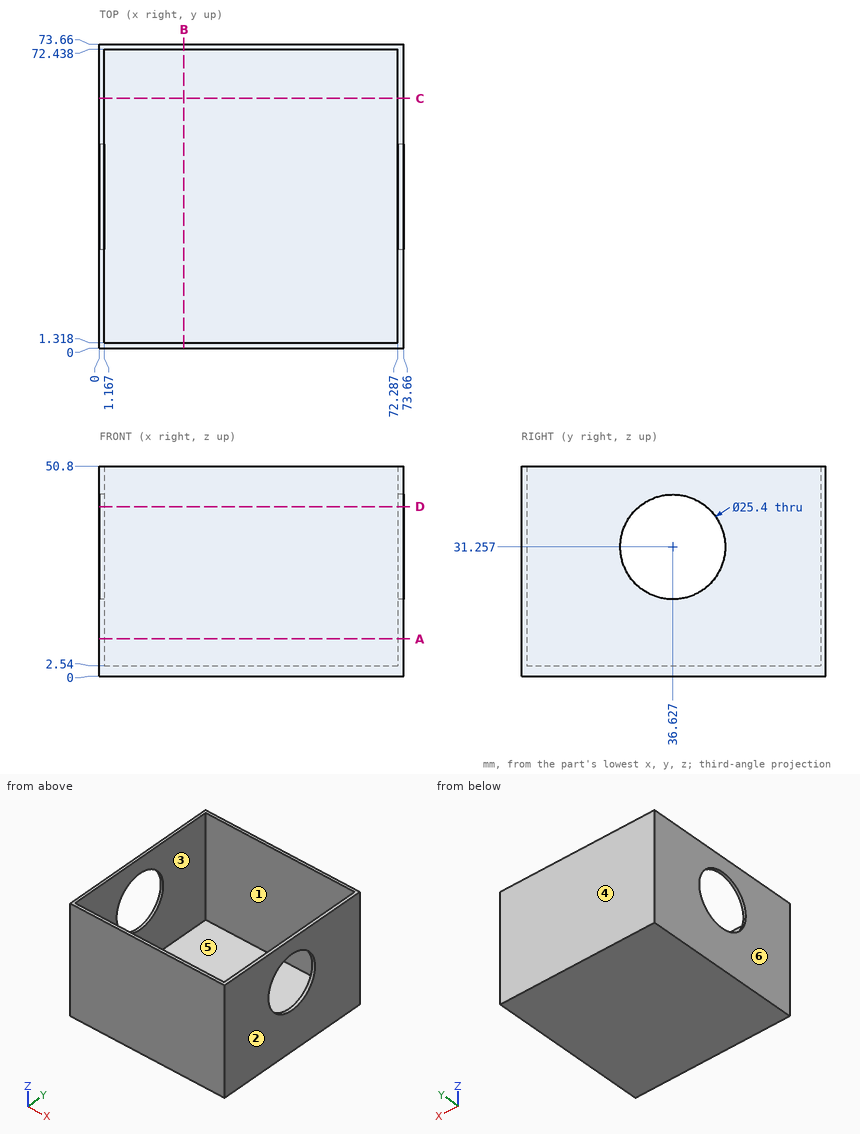
Drawing for the job (mm, zero at the part's lowest x, y, z). A direction names the side the tool comes from. Round coordinates to 2 decimals unless told otherwise and drop trailing zeros. Write each loop counter-clockwise with the first axis right and the second up, starting at its lowest first coordinate (ties: lowest second). Pieces come first, ordered by that corner, then holes. Notation, with made-up numbers: (4.5, 59.25) - (40.5, 59.25) arc R21 cw to (40.5, 79.25) - close; hole circle Ø11 at (67, 29). An arc over 180 degrees is marked (long way). Return JSON: item names as keys, results as strings. Group by question number.
Item 1: Band-saw the part on A-A on z = 9. List the corners of the cut face in (x, y).
Item 2: Flat gauge pin, fed straight in: pin 1 Ø4 at (x, y) = (31.5, 60.5) entering from +Z. Where does the tip first touch, or does it go through?
Item 3: Mould opens along Y. For the marked faces 1, 2, 3 and 4 say: +Y half, -Y half, draft (parallel to the pull), parting line (faces both ways), or undercut.
Item 4: Band-saw the part on D-D on z = 41. List the corners of the cut face in (x, y).
Item 5: Band-saw the part on B-B on x = 20.5. List the corners of the cut face in (y, z).
Item 6: 3-axis set-ups, long thin cutter, end or side, ignore diameter. For the marked faces 5 and 6: which of +Z, -Z, +X, -X, +Y, -Y reach the whole face in a straight line?
Item 7: Band-saw the part on C-C on y = 60.5. List the corners of the cut face in (x, z).
Item 8: Probe probe 1 along X at (y, z) = (44, 4); probe 2 along Y at (x, z) = (68, 37.5); probe 3 along Z at (x, y) = (69, 27). List the from-to ranges inside material, lowest first.
Resolved:
{
 "1": {"outline": "(0, 0) - (73.66, 0) - (73.66, 73.66) - (0, 73.66) - close; hole (1.17, 1.32) - (72.29, 1.32) - (72.29, 72.44) - (1.17, 72.44) - close"},
 "2": {"pin 1": "stops at z = 2.54"},
 "3": {"face 1": "undercut", "face 2": "draft", "face 3": "undercut", "face 4": "+Y half"},
 "4": {"outline": "(0, 0) - (73.66, 0) - (73.66, 28.48) - (72.29, 28.48) - (72.29, 1.32) - (1.17, 1.32) - (1.17, 28.48) - (0, 28.48) - close; (0, 44.77) - (1.17, 44.77) - (1.17, 72.44) - (72.29, 72.44) - (72.29, 44.77) - (73.66, 44.77) - (73.66, 73.66) - (0, 73.66) - close"},
 "5": {"outline": "(0, 0) - (73.66, 0) - (73.66, 50.8) - (72.44, 50.8) - (72.44, 2.54) - (1.32, 2.54) - (1.32, 50.8) - (0, 50.8) - close"},
 "6": {"face 5": "+Z", "face 6": "+Z, -Z, -X, +Y, -Y"},
 "7": {"outline": "(0, 0) - (73.66, 0) - (73.66, 50.8) - (72.29, 50.8) - (72.29, 2.54) - (1.17, 2.54) - (1.17, 50.8) - (0, 50.8) - close"},
 "8": {"probe 1": "x = 0 to 1.17, 72.29 to 73.66", "probe 2": "y = 0 to 1.32, 72.44 to 73.66", "probe 3": "z = 0 to 2.54"}
}
